```python
from build123d import *

# Parameters (mm, degrees)
SKETCH_1_R          = 2.1
EXTRUDE_1_DEPTH     = 3
CHAMFER_1_SIZE      = 25
SKETCH_4_R          = 1
CUT_EXTRUDE_1_DEPTH = 68.812240783
CUT_EXTRUDE_2_DEPTH = 68.812240783
CHAMFER_2_SIZE      = 4
FILLET_1_R          = 2
CHAMFER_3_SIZE      = 2


with BuildPart() as part:
    # 草图1 → 凸台-拉伸1 (new, symmetric)
    with BuildSketch(Plane(origin=(0, 0, 0), x_dir=(1, 0, 0), z_dir=(0, 1, 0))):
        Polygon((-8.6, 4.965212315), (-8.6, -4.965212315), (0, -9.93042463), (8.6, -4.965212315), (8.6, 4.965212315), (42.5, 4.965212315), (42.5, -52.5), (-42.5, -52.5), (-42.5, 4.965212315), align=None)
        with Locations(Location((-32.5, -42.5, 0), (0, 0, 270))):
            Circle(SKETCH_1_R, mode=Mode.SUBTRACT)
        with Locations(Location((32.5, -42.5, 0), (0, 0, 270))):
            Circle(SKETCH_1_R, mode=Mode.SUBTRACT)
    extrude(amount=EXTRUDE_1_DEPTH, both=True)

    # 倒角1
    chamfer_1_edges = [part.edges().sort_by_distance(p)[0] for p in [
        (42.5, 0, -4.965212315),
        (-42.5, 0, -4.965212315),
    ]]
    chamfer(chamfer_1_edges, length=CHAMFER_1_SIZE)

    # 草图4 → 切除-拉伸1 (cut, through all)
    with BuildSketch(Plane(origin=(0, 3, 0), x_dir=(1, 0, 0), z_dir=(0, 1, 0))):
        with Locations((0, -9.93042463)):
            Circle(SKETCH_4_R)
        with Locations((-8.1, -4.099186911)):
            Circle(SKETCH_4_R)
        with Locations((8.1, -4.099186911)):
            Circle(SKETCH_4_R)
    extrude(amount=-CUT_EXTRUDE_1_DEPTH, mode=Mode.SUBTRACT)

    # 草图3 → 切除-拉伸2 (cut, through all)
    with BuildSketch(Plane(origin=(0, 3, 0), x_dir=(1, 0, 0), z_dir=(0, 1, 0))):
        Polygon((-28.081928446, -16.93042463), (-34.5, -23.348496184), (-34.5, -29.186291501), (-19.186291501, -44.5), (19.186291501, -44.5), (34.5, -29.186291501), (34.5, -23.348496184), (28.081928446, -16.93042463), align=None)
    extrude(amount=-CUT_EXTRUDE_2_DEPTH, mode=Mode.SUBTRACT)

    # 倒角2
    chamfer_2_edges = [part.edges().sort_by_distance(p)[0] for p in [
        (42.5, 0, 52.5),
        (-42.5, 0, 52.5),
    ]]
    chamfer(chamfer_2_edges, length=CHAMFER_2_SIZE)

    # 圆角1
    fillet_1_edges = [part.edges().sort_by_distance(p)[0] for p in [
        (-28.081928446, 0, 16.93042463),
        (28.081928446, 0, 16.93042463),
        (34.5, 0, 23.348496184),
        (34.5, 0, 29.186291501),
        (19.186291501, 0, 44.5),
        (-19.186291501, 0, 44.5),
        (-34.5, 0, 29.186291501),
        (-34.5, 0, 23.348496184),
    ]]
    fillet(fillet_1_edges, radius=FILLET_1_R)

    # 倒角3
    chamfer_3_edges = [part.edges().sort_by_distance(p)[0] for p in [
        (-32.5, 3, 40.4),
        (32.5, 3, 40.4),
    ]]
    chamfer(chamfer_3_edges, length=CHAMFER_3_SIZE)


solid = part.part
```
Here's how the part is built. I have some questions about the finished solid (model axes, mm). A direction names the side the tool comes from. Give positions to 0.01 mm unless a question says otherwise; leave off trailing zeros. Write each loop counter-clockwise with the first axis right and the second up, starting at its lowest first coordinate (ties: lowest second). Pieces come first, ordered by that corner, then holes. Notation, with made-up numbers: (31, -37) -> (54, -37) arc R26 ccw to (54, -13) -> close; hole circle Ø7 at (11.25, 84.25). An arc over 180 degrees is marked (long way). Use one line per item in the form item = value.
1) If I drill on L1, parallel to Z at x = 0, y = -0.6; L2, parallel to X at y = -1, z = 35; L3, parallel to Z at x = 14.5, y = 1.5, over which ranges is the centre line in solid material (lowest first)? Write a range as [from, to].
Verdict:
L1 = [10.93, 16.93], [44.5, 52.5]
L2 = [-42.5, -28.69], [28.69, 42.5]
L3 = [-4.97, 16.93], [44.5, 52.5]
2) Suppose I cut it at D-D (z = 21). Please give me the cut outline in (x, y).
Verdict:
outline = (-42.5, -3) -> (-32.15, -3) -> (-32.15, 3) -> (-42.5, 3) -> close; (32.15, -3) -> (42.5, -3) -> (42.5, 3) -> (32.15, 3) -> close
3) I'm going to push flat-ended pins straight in: pin 1 (3 mm diameter, centred on y = -0.5, z = 0, fed in from -X); pin 2 (1.8 mm diameter, centred on y = 1, z = -1, fed in from +X). Where does each tip first touch, or does it pass through?
Verdict:
pin_1 = -23.97
pin_2 = 22.37
4) Suppose I cut it at A-A (x = 13). Please give me the cut outline in (y, z), and give its area (3 significant figures).
Verdict:
outline = (-3, -4.97) -> (3, -4.97) -> (3, 16.93) -> (-3, 16.93) -> close; (-3, 44.5) -> (3, 44.5) -> (3, 52.5) -> (-3, 52.5) -> close
area = 179 mm2
5) We'd pull the mould along Z, two halves only. Please class faces 4 (the face through (8.6, 0, -1)), 5 (the face through (-31.25, 0.04, 20.1)), 6 (the face through (1, 0, 52.5)): +Z half, -Z half, draft (parallel to the pull), parting line (faces both ways), or undercut.
Verdict:
face_4 = draft
face_5 = undercut
face_6 = +Z half
6) On a 3-axis mill with a long thin cutter (end or side, diameter ignored), from which of +Z, -Z, +X, -X, +Y, -Y can I reach the whole of each face in a straight line? I mean faces 1 (the face through (-8.6, 0, -1)), 2 (the face through (0, 0, 16.93)), 3 (the face through (-42.5, 0, 34)). Say none if no direction works.
Verdict:
face_1 = -Z, +Y, -Y
face_2 = +Y, -Y
face_3 = +Z, -Z, -X, +Y, -Y
7) Suppose I cut it at C-C (x = -32.5). Please give me the cut outline in (y, z), and give its area (3 significant figures).
Verdict:
outline = (-3, 10.03) -> (3, 10.03) -> (3, 21.35) -> (-3, 21.35) -> close; (-3, 31.19) -> (3, 31.19) -> (3, 38.4) -> (1, 40.4) -> (-3, 40.4) -> close; (-3, 44.6) -> (1, 44.6) -> (3, 46.6) -> (3, 52.5) -> (-3, 52.5) -> close
area = 167 mm2
8) Suppose I cut it at B-B (y = 2). Give the number of separate pieces and of enclosed holes in the cut face, and give its area (3 significant figures).
Verdict:
separate_pieces = 1
enclosed_holes = 3
area = 2,340 mm2
